Geometry check sheet. Reference: the model listing, model coordinates, mm. Face numbers are marked on the shaded views. A direction names the side the tool comes from. Round coordinates to 2 decimals unless told otherwise and drop trailing zeros. Order: outer loops, then holes, each group sorted by start corner. A loop starts at its lowest first (then second) coordinate and runs counter-clockwise, first axis right, second up.
(1) Set-up check for the marked faces 1 and 2: record each of +Z, -Z, +X, -X, +Y, -Y from which the full face is reachable in a straight line by a thin tool's end or side.
(2) Gauge pin test, flat end, axial feed: P1, Ø1.5, axis at x = 15, y = 26, coming from the +Z side. Record the tip position at first contact, or that the pin passes through.
(3) Cross-section at C-C on y = 16. Enter the section's corners in (x, z), and give its area (3 significant figures).
(4) Cross-section at A-A on z = 2. Enter the section's corners in (x, y), and give its area (3 significant figures).
(5) Cross-section at D-D on x = 5. Enter the section's corners in (y, z).
(6) Cross-section at B-B on x = 47. Enter the section's corners in (y, z), and give its area (3 significant figures).
(7) Thickness scan on L1, parallel to Y at x = 37, z = 6; L2, parallel to Y at x = 28, z = 7.25; L3, parallel to X at y = 28.5, z = 1.5. Record the ranges inside material, lowest first.
(8) Draft check along X on the marked faces 3, 4 and 5. Enter one of: pulls with the +X half, pulls with the -X half, needs draft (parallel to the pull), parting line crosses it, or undercut.
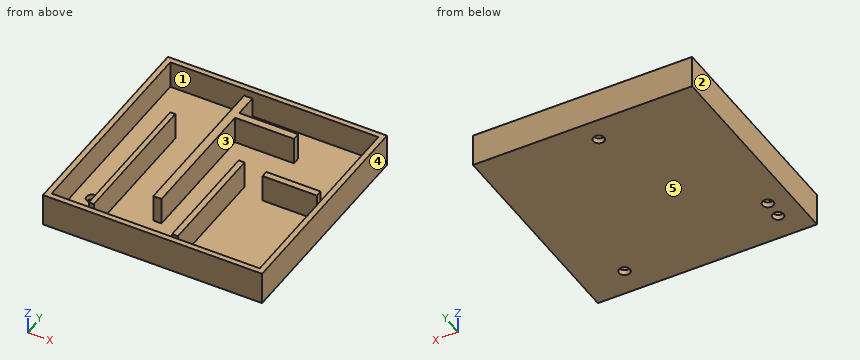
from build123d import *

# Parameters (mm, degrees)
F0_W     = 50.8
F0_H     = 50.8
F1_DEPTH = 7.62
F2_T     = -1.27
F3_W     = 1.152528
F3_H     = 33.115175
F3_W_2   = 13.665814
F3_H_2   = 1.731235
F3_W_3   = 1.353253
F3_H_3   = 27.104161
F3_W_4   = 12.571838
F3_H_4   = 1.511616
F4_DEPTH = 7.62
F5_R     = 1.27
F6_DEPTH = 7.621


with BuildPart() as f1:
    # F0 (on Top) → F1 (new body)
    with BuildSketch(Plane.XY):
        with Locations((25.4, 25.4)):
            Rectangle(F0_W, F0_H)
    extrude(amount=F1_DEPTH)

    # F2
    f2_openings = [f1.faces().sort_by_distance(p)[0] for p in [
        (25.4, 25.4, 7.62),
    ]]
    offset(amount=F2_T, openings=f2_openings)

    # F3 (on Top) → F4 (join)
    with BuildSketch(Plane.XY):
        with Locations((9.76058, 19.097683)):
            Rectangle(F3_W, F3_H)
        Polygon((21.372069, 42.3421), (21.372069, 47.670342), (19.46665, 47.670342), (19.46665, 10.718926), (21.372069, 10.718926), (21.372069, 40.610865), align=None)
        with Locations((28.204976, 41.476482)):
            Rectangle(F3_W_2, F3_H_2)
        with Locations((29.44033, 15.588485)):
            Rectangle(F3_W_3, F3_H_3)
        with Locations((41.71568, 27.930296)):
            Rectangle(F3_W_4, F3_H_4)
    extrude(amount=F4_DEPTH)

    # F5 (on Top) → F6 (cut, through all)
    with BuildSketch(Plane.XY):
        with Locations((5.450803, 6.229489)):
            Circle(F5_R)
        with Locations((5.256131, 10.706934)):
            Circle(F5_R)
        with Locations((41.075695, 6.229489)):
            Circle(F5_R)
        with Locations((24.723286, 45.358468)):
            Circle(F5_R)
    extrude(amount=F6_DEPTH, mode=Mode.SUBTRACT)


solid = f1.part
Found:
1. face 1: +Z
1. face 2: +Z, -Z, -X, +Y, -Y
2. P1: stops at z = 1.27
3. outline: (0, 0) - (50.8, 0) - (50.8, 7.62) - (49.53, 7.62) - (49.53, 1.27) - (30.12, 1.27) - (30.12, 7.62) - (28.76, 7.62) - (28.76, 1.27) - (21.37, 1.27) - (21.37, 7.62) - (19.47, 7.62) - (19.47, 1.27) - (10.34, 1.27) - (10.34, 7.62) - (9.18, 7.62) - (9.18, 1.27) - (1.27, 1.27) - (1.27, 7.62) - (0, 7.62) - close
3. area: 109 mm2
4. outline: (0, 0) - (50.8, 0) - (50.8, 50.8) - (0, 50.8) - close; (9.18, 2.54) - (10.34, 2.54) - (10.34, 35.66) - (9.18, 35.66) - close; (19.47, 10.72) - (21.37, 10.72) - (21.37, 40.61) - (35.04, 40.61) - (35.04, 42.34) - (21.37, 42.34) - (21.37, 47.67) - (19.47, 47.67) - close; (28.76, 2.04) - (30.12, 2.04) - (30.12, 29.14) - (28.76, 29.14) - close; (35.43, 27.17) - (48, 27.17) - (48, 28.69) - (35.43, 28.69) - close; hole (1.27, 1.27) - (49.53, 1.27) - (49.53, 49.53) - (1.27, 49.53) - close
4. area: 440 mm2
5. outline: (0, 0) - (5.04, 0) - (5.04, 1.27) - (1.27, 1.27) - (1.27, 7.62) - (0, 7.62) - close; (7.42, 0) - (9.46, 0) - (9.46, 1.27) - (7.42, 1.27) - close; (11.95, 0) - (50.8, 0) - (50.8, 7.62) - (49.53, 7.62) - (49.53, 1.27) - (11.95, 1.27) - close
6. outline: (0, 0) - (50.8, 0) - (50.8, 7.62) - (49.53, 7.62) - (49.53, 1.27) - (28.69, 1.27) - (28.69, 7.62) - (27.17, 7.62) - (27.17, 1.27) - (1.27, 1.27) - (1.27, 7.62) - (0, 7.62) - close
6. area: 90.2 mm2
7. L1: y = 0 to 1.27, 27.17 to 28.69, 49.53 to 50.8
7. L2: y = 0 to 1.27, 40.61 to 42.34, 49.53 to 50.8
7. L3: x = 0 to 1.27, 9.18 to 10.34, 19.47 to 21.37, 28.76 to 30.12, 35.43 to 48, 49.53 to 50.8
8. face 3: undercut
8. face 4: pulls with the +X half
8. face 5: needs draft
